```python
from build123d import *
from OCP.BRepFilletAPI import BRepFilletAPI_MakeChamfer

# Parameters (mm, degrees)
SKETCH1_W           = 76.2
SKETCH1_H           = 76.2
BOSS_EXTRUDE1_DEPTH = 25.4
SKETCH2_W           = 57.15
SKETCH2_H           = 57.15
CUT_EXTRUDE1_DEPTH  = 19.05
BOSS_EXTRUDE2_DEPTH = 12.7
CHAMFER1_SIZE       = 2.54
CHAMFER1_SIZE2      = 1.27
FILLET1_R           = 12.7
SKETCH4_W           = 33.02
SKETCH4_H           = 25.4
BOSS_EXTRUDE3_DEPTH = 48.26
CHAMFER2_SIZE       = 48.26
CHAMFER2_SIZE_2     = 10.16


with BuildPart() as part:
    # Sketch1 → Boss-Extrude1 (new body)
    with BuildSketch(Plane(origin=(0, 1478.617106037, 0), x_dir=(1, 0, 0), z_dir=(0, 1, 0))):
        with Locations((-492.049198231, -806.92955637)):
            Rectangle(SKETCH1_W, SKETCH1_H)
    extrude(amount=BOSS_EXTRUDE1_DEPTH)

    # Sketch2 → Cut-Extrude1 (cut)
    with BuildSketch(Plane(origin=(0, 1478.617106037, 0), x_dir=(-1, 0, 0), z_dir=(0, -1, 0))):
        with Locations((492.049198231, -806.92955637)):
            Rectangle(SKETCH2_W, SKETCH2_H)
    extrude(amount=-CUT_EXTRUDE1_DEPTH, mode=Mode.SUBTRACT)

    # Sketch3 → Boss-Extrude2 (add)
    with BuildSketch(Plane(origin=(0, 1478.617106037, 0), x_dir=(-1, 0, 0), z_dir=(0, -1, 0))):
        Polygon((530.149198231, -790.41955637), (527.482198231, -790.41955637), (527.482198231, -771.49655637), (508.559198231, -771.49655637), (508.559198231, -768.82955637), (530.149198231, -768.82955637), align=None)
        Polygon((530.149198231, -823.43955637), (527.482198231, -823.43955637), (527.482198231, -842.36255637), (508.559198231, -842.36255637), (508.559198231, -845.02955637), (530.149198231, -845.02955637), align=None)
        Polygon((475.539198231, -768.82955637), (475.539198231, -771.49655637), (456.616198231, -771.49655637), (456.616198231, -790.41955637), (453.949198231, -790.41955637), (453.949198231, -768.82955637), align=None)
        Polygon((475.539198231, -845.02955637), (475.539198231, -842.36255637), (456.616198231, -842.36255637), (456.616198231, -823.43955637), (453.949198231, -823.43955637), (453.949198231, -845.02955637), align=None)
    extrude(amount=BOSS_EXTRUDE2_DEPTH)

    # Chamfer1: one chamfer whose edges measure the first distance from different faces: ONE call of the kernel's chamfer builder (chamfer() names one face for all edges)
    chamfer1_edges_1 = [part.edges().sort_by_distance(p)[0] for p in [
        (-518.020698231, 1465.917106037, 771.49655637),
    ]]
    chamfer1_side_1 = [part.faces().sort_by_distance(p)[0] for p in [
        (-518.020698231, 1472.267106037, 771.49655637),
    ]]
    chamfer1_edges_2 = [part.edges().sort_by_distance(p)[0] for p in [
        (-527.482198231, 1465.917106037, 780.95805637),
    ]]
    chamfer1_side_2 = [part.faces().sort_by_distance(p)[0] for p in [
        (-527.482198231, 1472.267106037, 780.95805637),
    ]]
    chamfer1_edges_3 = [part.edges().sort_by_distance(p)[0] for p in [
        (-527.482198231, 1465.917106037, 832.90105637),
    ]]
    chamfer1_side_3 = [part.faces().sort_by_distance(p)[0] for p in [
        (-527.482198231, 1472.267106037, 832.90105637),
    ]]
    chamfer1_edges_4 = [part.edges().sort_by_distance(p)[0] for p in [
        (-518.020698231, 1465.917106037, 842.36255637),
    ]]
    chamfer1_side_4 = [part.faces().sort_by_distance(p)[0] for p in [
        (-518.020698231, 1472.267106037, 842.36255637),
    ]]
    chamfer1_edges_5 = [part.edges().sort_by_distance(p)[0] for p in [
        (-466.077698231, 1465.917106037, 771.49655637),
    ]]
    chamfer1_side_5 = [part.faces().sort_by_distance(p)[0] for p in [
        (-466.077698231, 1472.267106037, 771.49655637),
    ]]
    chamfer1_edges_6 = [part.edges().sort_by_distance(p)[0] for p in [
        (-456.616198231, 1465.917106037, 780.95805637),
    ]]
    chamfer1_side_6 = [part.faces().sort_by_distance(p)[0] for p in [
        (-456.616198231, 1472.267106037, 780.95805637),
    ]]
    chamfer1_edges_7 = [part.edges().sort_by_distance(p)[0] for p in [
        (-466.077698231, 1465.917106037, 842.36255637),
    ]]
    chamfer1_side_7 = [part.faces().sort_by_distance(p)[0] for p in [
        (-466.077698231, 1472.267106037, 842.36255637),
    ]]
    chamfer1_edges_8 = [part.edges().sort_by_distance(p)[0] for p in [
        (-456.616198231, 1465.917106037, 832.90105637),
    ]]
    chamfer1_side_8 = [part.faces().sort_by_distance(p)[0] for p in [
        (-456.616198231, 1472.267106037, 832.90105637),
    ]]
    chamfer1 = BRepFilletAPI_MakeChamfer(part.part.solid().wrapped)
    for e in chamfer1_edges_1:
        chamfer1.Add(CHAMFER1_SIZE, CHAMFER1_SIZE2, e.wrapped, chamfer1_side_1[0].wrapped)  # the first distance lies on this face
    for e in chamfer1_edges_2:
        chamfer1.Add(CHAMFER1_SIZE, CHAMFER1_SIZE2, e.wrapped, chamfer1_side_2[0].wrapped)  # the first distance lies on this face
    for e in chamfer1_edges_3:
        chamfer1.Add(CHAMFER1_SIZE, CHAMFER1_SIZE2, e.wrapped, chamfer1_side_3[0].wrapped)  # the first distance lies on this face
    for e in chamfer1_edges_4:
        chamfer1.Add(CHAMFER1_SIZE, CHAMFER1_SIZE2, e.wrapped, chamfer1_side_4[0].wrapped)  # the first distance lies on this face
    for e in chamfer1_edges_5:
        chamfer1.Add(CHAMFER1_SIZE, CHAMFER1_SIZE2, e.wrapped, chamfer1_side_5[0].wrapped)  # the first distance lies on this face
    for e in chamfer1_edges_6:
        chamfer1.Add(CHAMFER1_SIZE, CHAMFER1_SIZE2, e.wrapped, chamfer1_side_6[0].wrapped)  # the first distance lies on this face
    for e in chamfer1_edges_7:
        chamfer1.Add(CHAMFER1_SIZE, CHAMFER1_SIZE2, e.wrapped, chamfer1_side_7[0].wrapped)  # the first distance lies on this face
    for e in chamfer1_edges_8:
        chamfer1.Add(CHAMFER1_SIZE, CHAMFER1_SIZE2, e.wrapped, chamfer1_side_8[0].wrapped)  # the first distance lies on this face
    add(Compound.cast(chamfer1.Shape()), mode=Mode.REPLACE)

    # Fillet1
    fillet1_edges = [part.edges().sort_by_distance(p)[0] for p in [
        (-530.149198231, 1504.017106037, 806.92955637),
        (-492.049198231, 1504.017106037, 845.02955637),
        (-453.949198231, 1504.017106037, 806.92955637),
    ]]
    fillet(fillet1_edges, radius=FILLET1_R)

    # Sketch4 → Boss-Extrude3 (add)
    with BuildSketch(Plane(origin=(0, 0, 768.82955637), x_dir=(-1, 0, 0), z_dir=(0, 0, -1))):
        with Locations((492.049198231, 1491.317106037)):
            Rectangle(SKETCH4_W, SKETCH4_H)
    extrude(amount=BOSS_EXTRUDE3_DEPTH)

    # Chamfer2
    # the kernel refuses this chamfer: 48.26, 10.16 mm, written as the material it takes off along each edge
    with BuildSketch(Plane(origin=(-508.559198231, 1353.240682796, 720.56955637), x_dir=(-0.007929773045437122, 0, 0.9999685588554512), z_dir=(0, 1, 0))) as chamfer2_piece_1_section:
        Polygon((CHAMFER2_SIZE * 0.999968558855, CHAMFER2_SIZE * 0.00792977304544), (-CHAMFER2_SIZE_2 * 0.00792977304544, CHAMFER2_SIZE_2 * 0.999968558855), (0, 0), align=None)
    chamfer2_piece_1 = extrude(amount=276.152846481, mode=Mode.PRIVATE)
    chamfer2_piece_1 = split(chamfer2_piece_1, bisect_by=Plane(origin=(-505.671976228, 1491.317106037, 768.82955637), z_dir=(0, 0, -1)), keep=Keep.TOP, mode=Mode.PRIVATE)
    add(chamfer2_piece_1, mode=Mode.SUBTRACT)
    with BuildSketch(Plane(origin=(-350.16277499, 1478.617106037, 720.56955637), x_dir=(0, -0.007929773045437122, 0.9999685588554512), z_dir=(-1, 0, 0))) as chamfer2_piece_2:
        Polygon((CHAMFER2_SIZE * 0.999968558855, CHAMFER2_SIZE * 0.00792977304544), (-CHAMFER2_SIZE_2 * 0.00792977304544, CHAMFER2_SIZE_2 * 0.999968558855), (0, 0), align=None)
    extrude(amount=283.772846481, mode=Mode.SUBTRACT)
    with BuildSketch(Plane(origin=(-475.539198231, 1629.393529277, 720.56955637), x_dir=(0.007929773045437122, 0, 0.9999685588554512), z_dir=(0, -1, 0))) as chamfer2_piece_3_section:
        Polygon((CHAMFER2_SIZE * 0.999968558855, CHAMFER2_SIZE * 0.00792977304544), (-CHAMFER2_SIZE_2 * 0.00792977304544, CHAMFER2_SIZE_2 * 0.999968558855), (0, 0), align=None)
    chamfer2_piece_3 = extrude(amount=276.152846481, mode=Mode.PRIVATE)
    chamfer2_piece_3 = split(chamfer2_piece_3, bisect_by=Plane(origin=(-478.426420234, 1491.317106037, 768.82955637), z_dir=(0, 0, -1)), keep=Keep.TOP, mode=Mode.PRIVATE)
    add(chamfer2_piece_3, mode=Mode.SUBTRACT)


solid = part.part
```
For this review, take the finished solid that the model builds, in its own axes (mm). A direction names the side the tool comes from. Coordinates: 2 decimals unless noted, no trailing zeros. Order: outer loops, then holes, each group sorted by start corner. A loop starts at its lowest first (then second) coordinate and runs counter-clockwise, first axis right, second up. Notation, with made-up numbers: (-33.5, 18.5) -> (6.5, 18.5) arc R19 ccw to (6.5, 26.5) -> close; hole circle Ø10 at (38.5, 60.25). An arc over 180 degrees is marked (long way). Answer as CSV lines item,"result".
Q1. For faces 1 (the face through (-453.949, 1481, 807)), 2 (the face through (-455.972, 1467.169, 833.677)), 3 (the face through (-455, 1465.917, 839)), 4 (the face through (-465, 1485, 768.83)), 5 (the face through (-508.559, 1472, 770)), list the 3-axis set-ups (+Z, -Z, +X, -X, +Y, -Y) from which the entire face can be reached by the end or side of a thin tool; tool diameter is ignored.
Model answer:
face 1,"+Z, -Z, +X, +Y, -Y"
face 2,"-Y"
face 3,"+Z, -Z, +X, -X, -Y"
face 4,"-Z, +X, +Y, -Y"
face 5,"+Z, -Z, -Y"
Q2. We need section A-A (y = 1490). State the section outline as (x, z) points.
Model answer:
outline,"(-530.15, 768.83) -> (-508.56, 768.83) -> (-498.4, 720.57) -> (-485.7, 720.57) -> (-475.54, 768.83) -> (-453.95, 768.83) -> (-453.95, 845.03) -> (-530.15, 845.03) -> close; hole (-520.62, 778.35) -> (-463.47, 778.35) -> (-463.47, 835.5) -> (-520.62, 835.5) -> close"
Q3. We need section D-D (z = 783). State the section outline as (x, y) points.
Model answer:
outline,"(-530.15, 1465.92) -> (-528.75, 1465.92) -> (-527.48, 1468.46) -> (-527.48, 1478.62) -> (-520.62, 1478.62) -> (-520.62, 1497.67) -> (-463.47, 1497.67) -> (-463.47, 1478.62) -> (-456.62, 1478.62) -> (-456.62, 1468.46) -> (-455.35, 1465.92) -> (-453.95, 1465.92) -> (-453.95, 1491.32) arc R12.7 ccw to (-466.65, 1504.02) -> (-517.45, 1504.02) arc R12.7 ccw to (-530.15, 1491.32) -> close"
Q4. Draft analysis for pull direction Z (two halves, no side actions). For faces 6 (the face through (-519, 1485, 768.83)), 7 (the face through (-475.539, 1472, 844)), 8 (the face through (-458, 1478.617, 807)), state which applies: released by +Z, released by -Z, zero draft, split by the parting line, or undercut.
Model answer:
face 6,"released by -Z"
face 7,"zero draft"
face 8,"undercut"
Q5. Clearance check with flat-ended pins moving along their axes: pin 1 Ø12 at (x, z) = (-471.5, 800) entering from -Y; pin 2 Ø12 at (y, z) = (1473, 750.5) entering from -X; pin 3 Ø2 at (y, z) = (1496.5, 733) entering from -X; pin 4 Ø8 at (y, z) = (1491, 750.5) entering from -X. State where each tip first meets the part, or that it passes through.
Model answer:
pin 1,"stops at y = 1497.67"
pin 2,"passes through"
pin 3,"stops at x = -501.23"
pin 4,"stops at x = -505.54"
Q6. We need section C-C (x = -510). State the section outline as (y, z) points.
Model answer:
outline,"(1465.92, 768.83) -> (1504.02, 768.83) -> (1504.02, 832.33) arc R12.7 ccw to (1491.32, 845.03) -> (1465.92, 845.03) -> (1465.92, 843.63) -> (1468.46, 842.36) -> (1478.62, 842.36) -> (1478.62, 835.5) -> (1497.67, 835.5) -> (1497.67, 778.35) -> (1478.62, 778.35) -> (1478.62, 771.5) -> (1468.46, 771.5) -> (1465.92, 770.23) -> close"
Q7. Wall thickness on line 1 along X through (y, z) = (1469.5, 770.5); line 2 along X through (y, z) = (1482, 835); line 3 along Z through (x, y) = (-463.5, 1469): over which ranges is each line inside the solid? List them lowest first. Write a range as [from, to].
Model answer:
line 1,"x = [-530.15, -508.56], [-475.54, -453.95]"
line 2,"x = [-530.15, -520.62], [-463.47, -453.95]"
line 3,"z = [768.83, 771.5], [842.36, 845.03]"
Q8. We need section B-B (y = 1471). State the section outline as (x, z) points.
Model answer:
outline,"(-530.15, 768.83) -> (-508.56, 768.83) -> (-508.56, 771.5) -> (-527.48, 771.5) -> (-527.48, 790.42) -> (-530.15, 790.42) -> close; (-530.15, 823.44) -> (-527.48, 823.44) -> (-527.48, 842.36) -> (-508.56, 842.36) -> (-508.56, 845.03) -> (-530.15, 845.03) -> close; (-475.54, 768.83) -> (-453.95, 768.83) -> (-453.95, 790.42) -> (-456.62, 790.42) -> (-456.62, 771.5) -> (-475.54, 771.5) -> close; (-475.54, 842.36) -> (-456.62, 842.36) -> (-456.62, 823.44) -> (-453.95, 823.44) -> (-453.95, 845.03) -> (-475.54, 845.03) -> close"
